Study the drawing (mm; zero at the part's minimum x, y, z) and answer. Give positions to 0.01 mm unless a question says otherwise; leave off trailing zeros. Order: outer loops, then holes, each group sorted by start corner. A loop starts at its lowest first (then second) coordinate and runs counter-clockwise, first axis right, second up.
Item 1: A cutting plane is placed at A-A (y = 353.5). Write down the section's boundary in (x, z).
Item 2: A cutting plane is placed at C-C (x = 154.5). Write down the section's boundary in (y, z).
Item 3: Find the intervals of material crossed by line 1 along X through (y, z) = (361, 5.25); line 2 along Y through (x, z) = (241, 1.25); line 3 along Y through (x, z) = (159, 11.5), in increasing order.
Item 4: A cutting plane is placed at B-B (z = 4). Write down the section's boundary in (x, y).
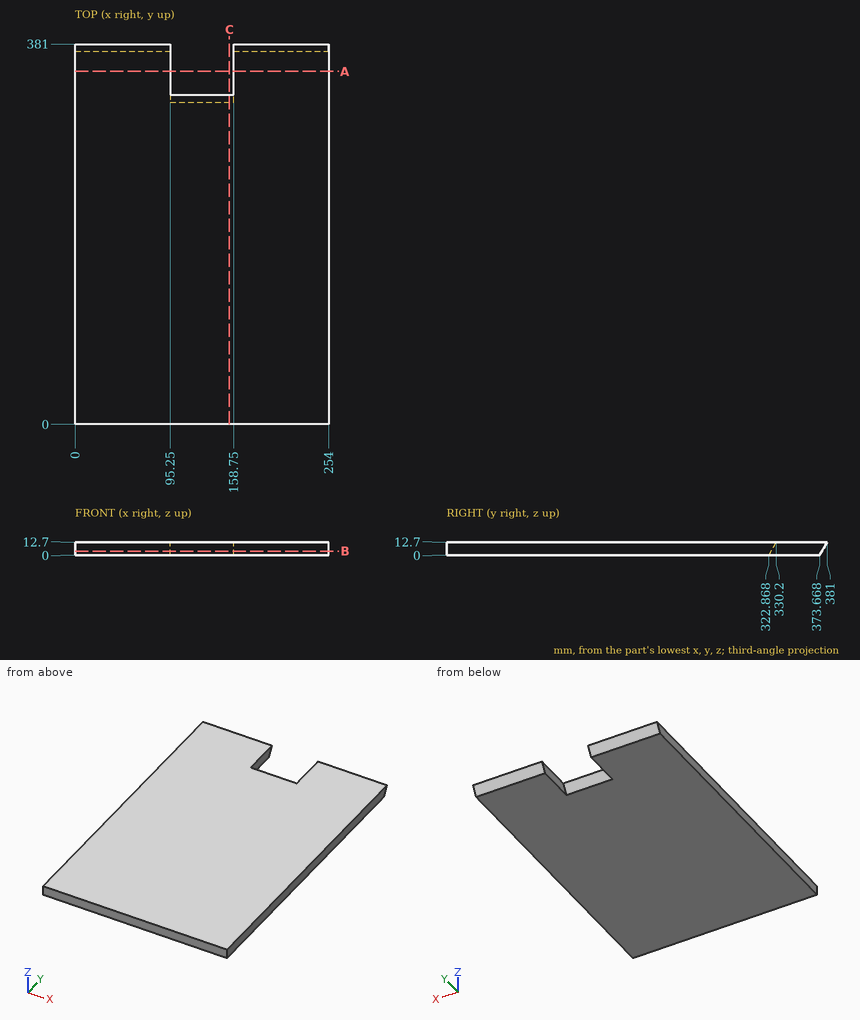
Response values:
1. outline: (0, 0) - (95.25, 0) - (95.25, 12.7) - (0, 12.7) - close; (158.75, 0) - (254, 0) - (254, 12.7) - (158.75, 12.7) - close
2. outline: (0, 0) - (322.87, 0) - (330.2, 12.7) - (0, 12.7) - close
3. line 1: x = 0 to 95.25, 158.75 to 254
3. line 2: y = 0 to 374.39
3. line 3: y = 0 to 380.31
4. outline: (0, 0) - (254, 0) - (254, 375.98) - (158.75, 375.98) - (158.75, 325.18) - (95.25, 325.18) - (95.25, 375.98) - (0, 375.98) - close
